Check sheet for the modelled part. Datum: model origin and axes. Units: mm. Round coordinates to 2 decimals unless told otherwise and drop trailing zeros. Order: outer loops, then holes, each group sorted by start corner. A loop starts at its lowest first (then second) coordinate and runs counter-clockwise, first axis right, second up.
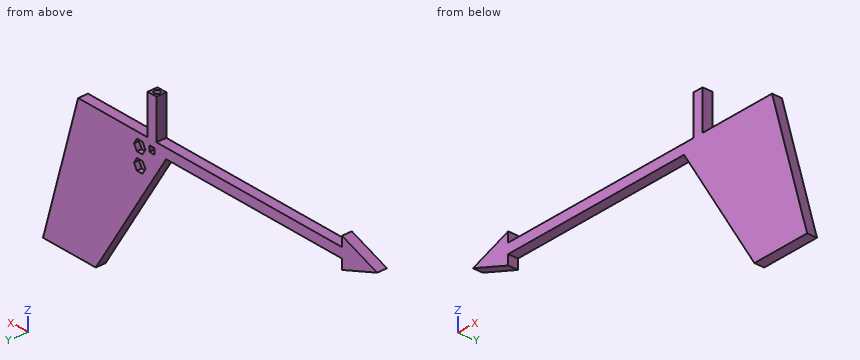
```python
from build123d import *

# Parameters (mm, degrees)
BOSS_EXTRUDE1_DEPTH = 2.5
CUT_EXTRUDE2_DEPTH  = 2.5
SKETCH3_W           = 5
SKETCH3_H           = 5
BOSS_EXTRUDE2_DEPTH = 20
SKETCH4_R           = 1.5
CUT_EXTRUDE3_DEPTH  = 23
SKETCH6_W           = 3
SKETCH6_H           = 3
CUT_EXTRUDE5_DEPTH  = 4


with BuildPart() as part:
    # Sketch1 → Boss-Extrude1 (new, symmetric)
    with BuildSketch(Plane(origin=(0, 0, 0), x_dir=(1, 0, 0), z_dir=(0, 1, 0))):
        Polygon((-20, 0), (0, 7.5), (0, 2.5), (100, 2.5), (140, 67.5), (170, 67.5), (150, -2.5), (0, -2.5), (0, -7.5), align=None)
    extrude(amount=BOSS_EXTRUDE1_DEPTH, both=True)

    # Sketch2 → Cut-Extrude2 (cut)
    with BuildSketch(Plane(origin=(0, 2.5, 0), x_dir=(1, 0, 0), z_dir=(0, 1, 0))):
        Polygon((118.233161507, 12), (116.616580754, 14.8), (113.383419246, 14.8), (111.766838493, 12), (113.383419246, 9.2), (116.616580754, 9.2), align=None)
        Polygon((118.233161507, 3.5), (116.616580754, 6.3), (113.383419246, 6.3), (111.766838493, 3.5), (113.383419246, 0.7), (116.616580754, 0.7), align=None)
    extrude(amount=-CUT_EXTRUDE2_DEPTH, mode=Mode.SUBTRACT)

    # Sketch3 → Boss-Extrude2 (add)
    with BuildSketch(Plane.XY.offset(2.5)):
        with Locations((108, 0)):
            Rectangle(SKETCH3_W, SKETCH3_H)
    extrude(amount=BOSS_EXTRUDE2_DEPTH)

    # Sketch4 → Cut-Extrude3 (cut)
    with BuildSketch(Plane.XY.offset(22.5)):
        with Locations((108, 0)):
            Circle(SKETCH4_R)
    extrude(amount=-CUT_EXTRUDE3_DEPTH, mode=Mode.SUBTRACT)

    # Sketch6 → Cut-Extrude5 (cut)
    with BuildSketch(Plane(origin=(0, 2.5, 0), x_dir=(1, 0, 0), z_dir=(0, 1, 0))):
        with Locations((108, 2)):
            Rectangle(SKETCH6_W, SKETCH6_H)
    extrude(amount=-CUT_EXTRUDE5_DEPTH, mode=Mode.SUBTRACT)


solid = part.part
```
Item 1: Sectioned sample at B-B (z = -19). Record the cut outline in (x, y), and give its area (3 significant figures).
Answer:
outline: (110.15, -2.5) - (156.14, -2.5) - (156.14, 2.5) - (110.15, 2.5) - close
area: 230 mm2
Item 2: Sectioned sample at A-A (x = 95). Record the cut outline in (y, z).
Answer:
outline: (-2.5, -2.5) - (2.5, -2.5) - (2.5, 2.5) - (-2.5, 2.5) - close
Item 3: Scan lines: line 1 along Y through (x, z) = (108, 16); line 2 along Z through (x, y) = (69.5, 1.1); line 3 along X through (y, z) = (-1.25, 17). Record each from-to range of solid material in increasing order.
Answer:
line 1: y = -2.5 to -1.5, 1.5 to 2.5
line 2: z = -2.5 to 2.5
line 3: x = 105.5 to 107.17, 108.83 to 110.5
Item 4: Go/stop test with flat-tipped pins: P1, Ø1, axis at x = 48.5, y = 2, coming from the -Z side; P2, Ø4.5, axis at x = 115.5, z = -5, coming from the +Y side; P3, Ø0.8, axis at x = 115.5, y = 1.5, coming from the +Z side; P4, Ø0.8, axis at x = 114.5, y = 1.5, coming from the -Z side. Record where each tip stops, or that it passes through.
Answer:
P1: stops at z = -2.5
P2: stops at y = 2.5
P3: stops at z = 2.5
P4: stops at z = -26.71
